Could you check a few things on this model? Use its own coordinates, in mm. Give positions to 0.01 mm unless a question says otherwise; leave off trailing zeros. Loops run counter-clockwise (first coordinate to the right, second up) from the corner with the lowest first, then second, coordinate; pieces in that order, holes last. Notation, with made-up numbers: M -32,72 L 20,72 A13 cw 20,96 Z; hole C -36.5,86 d11. An arc over 180 degrees is marked long. Use a Markdown table: item, result. Add a question column.
1) Will these pins go through, and if not, where does the flat tip stop? pin 1 Ø3.5 at (x, y) = (-50.8, 101.6) entering from +Z; pin 2 Ø1 at (x, z) = (-3, 3) entering from +Y; pin 3 Ø1 at (x, z) = (-52, 2.5) entering from -Y.
2) Suppose I cut it at C-C on z = 1.5. List the corners of the cut face in (x, y) for me (3 decimals), and give its area (3 significant figures).
3) If I drill on line 1 along Y through (x, z) = (-50.8, 2.5); line 2 along Y through (x, z) = (0, 3); line 3 along Y through (x, z) = (-2, 6), over which ranges is the centre line in solid material (lowest first)? Write a range as [from, to].
4) Suppose I cut it at D-D on x = 0. List the corners of the cut face in (y, z) for me, and give its area (3 significant figures).
5) Suppose I cut it at A-A on x = -50.8. List the corners of the cut face in (y, z) for me, and give its area (3 significant figures).
6) Suppose I cut it at B-B on y = 101.6. List the corners of the cut face in (x, z) for me, and give its area (3 significant figures).
```python
from build123d import *

# Parameters (mm, degrees)
BOSS_EXTRUDE1_DEPTH      = 6.35
FILLET1_R                = 3.175
M5_CLEARANCE_HOLE1_D     = 5.5
M5_CLEARANCE_HOLE1_DEPTH = 18.75
M5_CLEARANCE_HOLE1_TIP   = 1.652366702


with BuildPart() as part:
    # Sketch1 → Boss-Extrude1 (new body)
    with BuildSketch(Plane.XY):
        Polygon((-12.7, 29.029487758), (-12.7, 58.239487758), (-43.360512242, 88.9), (-81.460512242, 88.9), (-81.460512242, 114.3), (-32.839487758, 114.3), (12.7, 68.760512242), (12.7, 37.919487758), (12.7, 29.029487758), (12.7, 20.139487758), (-12.7, 20.139487758), align=None)
    extrude(amount=BOSS_EXTRUDE1_DEPTH)

    # Fillet1
    fillet1_edges = [part.edges().sort_by_distance(p)[0] for p in [
        (-12.7, 58.239487758, 3.175),
        (-43.360512242, 88.9, 3.175),
    ]]
    fillet(fillet1_edges, radius=FILLET1_R)

    # M5 Clearance Hole1
    with Locations(Plane.XY.offset(6.35)):
        with Locations((0, 50.8), (-50.8, 101.6), (-68.760512242, 101.6), (0, 32.839487758)):
            Hole(M5_CLEARANCE_HOLE1_D / 2, depth=M5_CLEARANCE_HOLE1_DEPTH)
            with Locations((0, 0, -(M5_CLEARANCE_HOLE1_DEPTH + M5_CLEARANCE_HOLE1_TIP / 2))):  # 118° drill point
                Cone(0, M5_CLEARANCE_HOLE1_D / 2, M5_CLEARANCE_HOLE1_TIP, mode=Mode.SUBTRACT)


solid = part.part
```
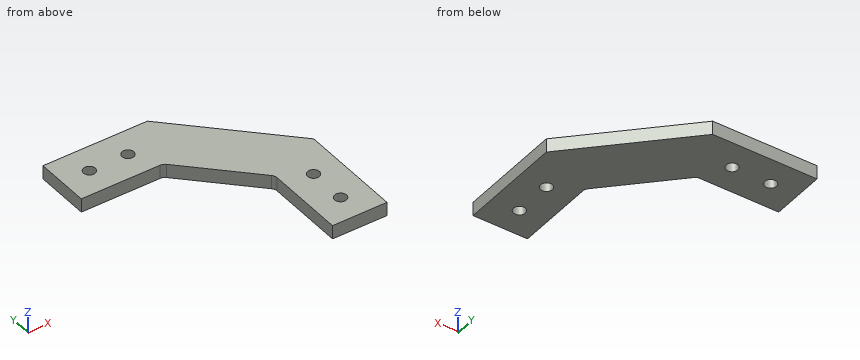
Answer block:
| question | item | result |
|---|---|---|
| 1 | pin 1 | passes through |
| 1 | pin 2 | stops at y = 84.96 |
| 1 | pin 3 | stops at y = 88.9 |
| 2 | outline | M -81.461,88.9 L -44.676,88.9 A3.175 cw -42.431,87.97 L -13.63,59.169 A3.175 cw -12.7,56.924 L -12.7,20.139 L 12.7,20.139 L 12.7,68.761 L -32.839,114.3 L -81.461,114.3 Z; hole C -68.761,101.6 d5.5; hole C -50.8,101.6 d5.5; hole C 0,32.839 d5.5; hole C 0,50.8 d5.5 |
| 2 | area | 3,480 mm^2 |
| 3 | line 1 | y = [88.9, 98.85], [104.35, 114.3] |
| 3 | line 2 | y = [20.14, 30.09], [35.59, 48.05], [53.55, 81.46] |
| 3 | line 3 | y = [20.14, 30.95], [34.73, 48.91], [52.69, 83.46] |
| 4 | outline | M 20.14,0 L 30.09,0 L 30.09,6.35 L 20.14,6.35 Z; M 35.59,0 L 48.05,0 L 48.05,6.35 L 35.59,6.35 Z; M 53.55,0 L 81.46,0 L 81.46,6.35 L 53.55,6.35 Z |
| 4 | area | 320 mm^2 |
| 5 | outline | M 88.9,0 L 98.85,0 L 98.85,6.35 L 88.9,6.35 Z; M 104.35,0 L 114.3,0 L 114.3,6.35 L 104.35,6.35 Z |
| 5 | area | 126 mm^2 |
| 6 | outline | M -81.46,0 L -71.51,0 L -71.51,6.35 L -81.46,6.35 Z; M -66.01,0 L -53.55,0 L -53.55,6.35 L -66.01,6.35 Z; M -48.05,0 L -20.14,0 L -20.14,6.35 L -48.05,6.35 Z |
| 6 | area | 320 mm^2 |
